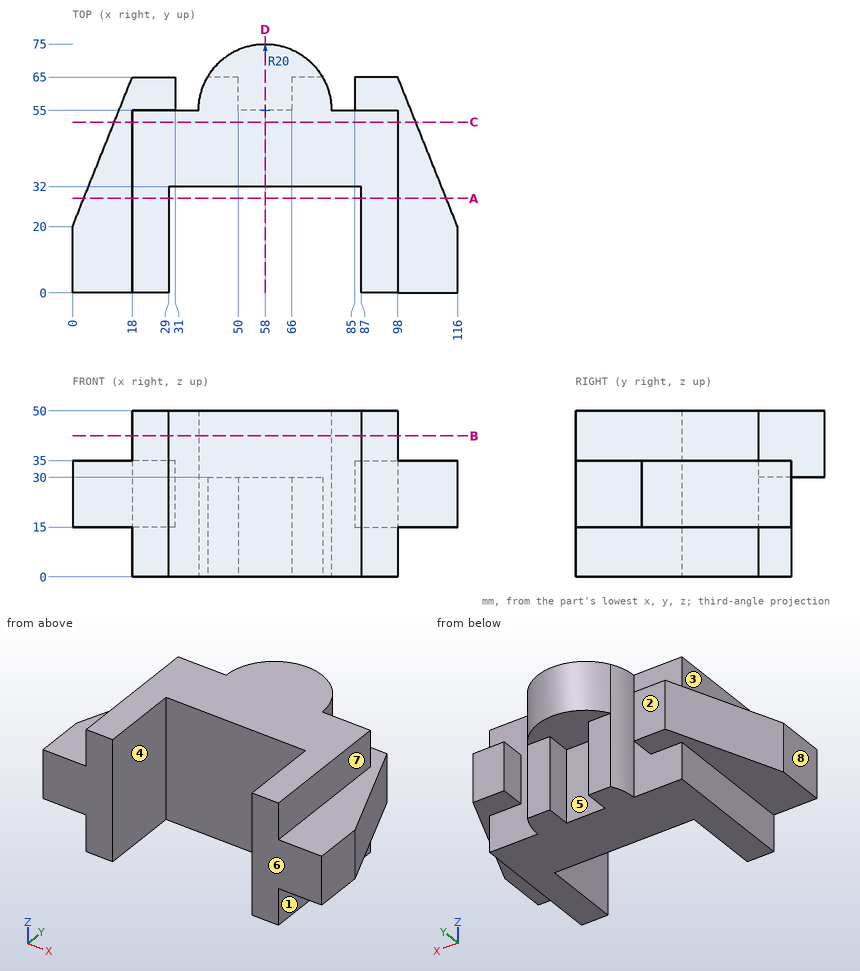
Check sheet for the drawn part. Datum: minimum x, y, z corner. Units: mm. A direction names the side the tool comes from. Round coordinates to 2 decimals unless told otherwise and drop trailing zeros. Loops run counter-clockwise (first coordinate to the right, second up) from the corner with the lowest first, then second, coordinate; pieces in that order, holes last.
Item 1: Thickness scan on line 1 (X direction, y = 19, z = 4); line 2 (X direction, y = 60, z = 19); line 3 (X direction, y = 57.5, z = 24.5). Record the ranges inside material, lowest first.
Item 2: Cross-section at C-C on y = 51.5. Record the boundary of the cut face in (x, z), then the cut area to 3 significant figures.
Item 3: Cross-section at B-B on z = 42.5. Record the boundary of the cut face in (x, y), then the cut area to 3 significant figures.
Item 4: Access from +Z, -Z, +X, -X, +Y, -Y to the whole of each face (thin tool, end or side, straight path). Record for the marked faces 1, 2, 3 and 4.
Item 5: Cross-section at A-A on y = 28.5. Record the boundary of the cut face in (x, z), then the cut area to 3 significant figures.
Item 6: Mould release check, pull along X, two halves, no side actions. Record for the marked faces 5, 6, 7 and 8: pulls with the +X half, pulls with the -X half, needs draft (parallel to the pull), parting line crosses it, or undercut.
Item 7: Cross-section at D-D on x = 58. Record the boundary of the cut face in (y, z), then the cut area to 3 significant figures.
Item 8: Gauge pin test, flat ends, axial feed: pin 1 (9.5 mm diameter, centred on y = 10, z = 29.5, fed in from -X); pin 2 (5 mm diameter, centred on y = 60, z = 18.5, fed in from -X); pin 3 (4.5 mm diameter, centred on y = 28.5, z = 6, fed in from +X); pin 4 (6 mm diameter, centred on x = 64, z = 24.5, fed in from +Y). Record the tip position at first contact, or that the pin passes through.
Answer sheet:
1. line 1: x = 18 to 29, 87 to 98
1. line 2: x = 16 to 31, 38.64 to 50, 66 to 77.36, 85 to 100
1. line 3: x = 15 to 31, 38.16 to 50, 66 to 77.84, 85 to 101
2. outline: (12.6, 15) - (18, 15) - (18, 0) - (98, 0) - (98, 15) - (103.4, 15) - (103.4, 35) - (98, 35) - (98, 50) - (18, 50) - (18, 35) - (12.6, 35) - close
2. area: 4,220 mm2
3. outline: (18, 0) - (29, 0) - (29, 32) - (87, 32) - (87, 0) - (98, 0) - (98, 55) - (78, 55) arc R20 ccw to (38, 55) - (18, 55) - close
3. area: 3,170 mm2
4. face 1: -Z, +X, +Y, -Y
4. face 2: +Z, -Z, -X, +Y
4. face 3: +Z, -X, +Y, -Y
4. face 4: +Z, -Z, -Y
5. outline: (3.4, 15) - (18, 15) - (18, 0) - (29, 0) - (29, 50) - (18, 50) - (18, 35) - (3.4, 35) - close; (87, 0) - (98, 0) - (98, 15) - (112.6, 15) - (112.6, 35) - (98, 35) - (98, 50) - (87, 50) - close
5. area: 1,680 mm2
6. face 5: undercut
6. face 6: needs draft
6. face 7: pulls with the +X half
6. face 8: pulls with the -X half
7. outline: (32, 0) - (55, 0) - (55, 30) - (75, 30) - (75, 50) - (32, 50) - close
7. area: 1,550 mm2
8. pin 1: stops at x = 0
8. pin 2: stops at x = 15
8. pin 3: stops at x = 98
8. pin 4: stops at y = 65
